Check sheet for the modelled part. Datum: model origin and axes. Units: mm. A direction names the side the tool comes from. Round coordinates to 2 decimals unless told otherwise and drop trailing zeros. Order: outer loops, then holes, each group sorted by start corner. A loop starts at its lowest first (then second) coordinate and runs counter-clockwise, first axis right, second up.
```python
from build123d import *

# Parameters (mm, degrees)
FILLET_R     = 0.2
POCKET_DEPTH = 1.3
FILLET001_R  = 0.2


with BuildPart() as part:
    # Sketch → Revolution (revolve)
    with BuildSketch(Plane.XY):
        Polygon((0, 0), (0, 42), (2.7, 42), (2.7, 40), (1.5, 40), (1.5, 0), align=None)
    revolve(axis=Axis((0, 0, 0), (0, 1, 0)))

    # Fillet
    fillet_edges = [part.edges().sort_by_distance(p)[0] for p in [
        (-2.7, 40, 0),
        (-2.7, 42, 0),
    ]]
    fillet(fillet_edges, radius=FILLET_R)

    # Sketch001 (on Face1 of Fillet) → Pocket (cut)
    with BuildSketch(Plane(origin=(0, 42, 0), x_dir=(-1, 0, 0), z_dir=(0, 1, 0))):
        Polygon((0.5, 1.5), (0.5, 0.5), (1.5, 0.5), (1.5, -0.5), (0.5, -0.5), (0.5, -1.5), (-0.5, -1.5), (-0.5, -0.5), (-1.5, -0.5), (-1.5, 0.5), (-0.5, 0.5), (-0.5, 1.5), align=None)
    extrude(amount=-POCKET_DEPTH, mode=Mode.SUBTRACT)

    # Fillet001
    fillet001_edges = [part.edges().sort_by_distance(p)[0] for p in [
        (0, 42, -1.5),
        (0.5, 42, -1),
        (1, 42, -0.5),
        (1.5, 42, 0),
        (1, 42, 0.5),
        (0.5, 42, 1),
        (-0.5, 42, 1),
        (0, 42, 1.5),
        (-1.5, 42, 0),
        (-1, 42, -0.5),
        (-0.5, 42, -1),
    ]]
    fillet(fillet001_edges, radius=FILLET001_R)


solid = part.part
```
Item 1: Sectioned sample at A-A (z = 0). Record the cut outline in (x, y), and give its area (3 significant figures).
Answer:
outline: (-2.7, 40.2) arc R0.2 ccw to (-2.5, 40) - (-1.5, 40) - (-1.5, 0) - (1.5, 0) - (1.5, 40) - (2.5, 40) arc R0.2 ccw to (2.7, 40.2) - (2.7, 41.8) arc R0.2 ccw to (2.5, 42) - (1.7, 42) arc R0.2 ccw to (1.5, 41.8) - (1.5, 40.7) - (-1.5, 40.7) - (-1.5, 41.8) arc R0.2 ccw to (-1.7, 42) - (-2.5, 42) arc R0.2 ccw to (-2.7, 41.8) - close
area: 127 mm2
Item 2: Go/stop test with flat-tipped pins: P1, Ø0.5, axis at y = 41, z = 1, coming from the +X side; P2, Ø1.1, axis at x = 1, y = 41.5, coming from the +Z side; P3, Ø0.8, axis at x = 1, y = 41.5, coming from the -Z side. Record where each tip stops, or that it passes through.
Answer:
P1: stops at x = 2.59
P2: stops at z = 2.66
P3: stops at z = -2.63
Item 3: Scan lines: line 1 along Y through (x, z) = (1.65, -1.1); line 2 along Y through (x, z) = (0.65, -0.05); line 3 along X through (y, z) = (25, -0.1). Record each from-to range of solid material in increasing order.
Answer:
line 1: y = 40 to 42
line 2: y = 0 to 40.7
line 3: x = -1.5 to 1.5
Item 4: Sectioned sample at B-B (x = 0). Record the cut outline in (y, z).
Answer:
outline: (0, -1.5) - (40, -1.5) - (40, -2.5) arc R0.2 ccw to (40.2, -2.7) - (41.8, -2.7) arc R0.2 ccw to (42, -2.5) - (42, -1.7) arc R0.2 ccw to (41.8, -1.5) - (40.7, -1.5) - (40.7, 1.5) - (41.8, 1.5) arc R0.2 ccw to (42, 1.7) - (42, 2.5) arc R0.2 ccw to (41.8, 2.7) - (40.2, 2.7) arc R0.2 ccw to (40, 2.5) - (40, 1.5) - (0, 1.5) - close
Item 5: Sectioned sample at C-C (y = 6). Record the cut outline in (x, z), and give its area (3 significant figures).
Answer:
outline: circle Ø3 at (0, 0)
area: 7.07 mm2
Item 6: Access from +Z, -Z, +X, -X, +Y, -Y to the whole of each face (thin tool, end or side, straight path). Record for faces 1 (the flat face through (-1, 42, 1)), 2 (the flat face through (-0.5, 41, -1)), 3 (the flat face through (2, 40, 0)).
Answer:
face 1: +Z, -Z, +X, -X, +Y
face 2: +Y
face 3: -Y
Item 7: Release check for a two-part mould opening along Z. For faces 4 (the flat face through (0, 0, 0)), 5 (the cylindrical face through (-0.585, 40.989, 2.636)), 6 (the flat face through (-0.5, 41, 1)), 7 (the flat face through (-1, 41, 0.5)) record: released by +Z, released by -Z, zero draft, split by the parting line, or undercut.
Answer:
face 4: zero draft
face 5: split by the parting line
face 6: undercut
face 7: undercut
